```python
from build123d import *

# Parameters (mm, degrees)
SKETCH1_W           = 6.5
SKETCH1_H           = 6.5
SKETCH1_R           = 1.5
BOSS_EXTRUDE1_DEPTH = 5.8
SKETCH2_W           = 6.5
SKETCH2_H           = 5.8
BOSS_EXTRUDE2_DEPTH = 8.85
SKETCH6_W           = 8.85
SKETCH6_H           = 5.8
BOSS_EXTRUDE6_DEPTH = 12.06
SKETCH7_W           = 6.5
SKETCH7_H           = 8.85
BOSS_EXTRUDE7_DEPTH = 75.25
BOSS_EXTRUDE8_DEPTH = 8.85
FILLET3_R           = 20
SKETCH10_R          = 1.125
CUT_EXTRUDE1_DEPTH  = 84.899470201
CUT_EXTRUDE2_START  = -2
SKETCH11_R          = 1.125
CUT_EXTRUDE2_DEPTH  = 2
SKETCH13_W          = 12.06
SKETCH13_H          = 0.25
CUT_EXTRUDE4_DEPTH  = 84.36611182
SKETCH14_W          = 6.5
SKETCH14_H          = 0.25
CUT_EXTRUDE5_DEPTH  = 78.739105989


with BuildPart() as part:
    # Sketch1 → Boss-Extrude1 (new body)
    with BuildSketch(Plane(origin=(0, 0, 0), x_dir=(1, 0, 0), z_dir=(0, 1, 0))):
        Rectangle(SKETCH1_W, SKETCH1_H)
        with Locations(Location((0, 0, 0), (0, 0, 270))):
            Circle(SKETCH1_R, mode=Mode.SUBTRACT)
    extrude(amount=BOSS_EXTRUDE1_DEPTH)

    # Sketch2 → Boss-Extrude2 (add)
    with BuildSketch(Plane.XY.offset(3.25)):
        with Locations((0, 2.9)):
            Rectangle(SKETCH2_W, SKETCH2_H)
    extrude(amount=BOSS_EXTRUDE2_DEPTH)

    # Sketch6 → Boss-Extrude6 (add)
    with BuildSketch(Plane(origin=(3.25, 0, 0), x_dir=(0, 0, -1), z_dir=(1, 0, 0))):
        with Locations((-7.675, 2.9)):
            Rectangle(SKETCH6_W, SKETCH6_H)
    extrude(amount=BOSS_EXTRUDE6_DEPTH)

    # Sketch7 → Boss-Extrude7 (add)
    with BuildSketch(Plane(origin=(0, 5.8, 0), x_dir=(1, 0, 0), z_dir=(0, 1, 0))):
        with Locations((12.06, -7.675)):
            Rectangle(SKETCH7_W, SKETCH7_H)
    extrude(amount=BOSS_EXTRUDE7_DEPTH)

    # Sketch8 → Boss-Extrude8 (add)
    with BuildSketch(Plane.XY.offset(12.1)):
        Polygon((-3.25, 5.8), (8.81, 5.8), (8.81, 17.86), align=None)
    extrude(amount=-BOSS_EXTRUDE8_DEPTH)

    # Fillet3
    fillet3_edges = [part.edges().sort_by_distance(p)[0] for p in [
        (8.81, 17.86, 7.675),
    ]]
    fillet(fillet3_edges, radius=FILLET3_R)

    # Sketch10 → Cut-Extrude1 (cut, through all)
    with BuildSketch(Plane.XY.offset(12.1)):
        with Locations((12.06, 77.25)):
            Circle(SKETCH10_R)
        with Locations((12.06, 40.05)):
            Circle(SKETCH10_R)
    extrude(amount=-CUT_EXTRUDE1_DEPTH, mode=Mode.SUBTRACT)

    # Sketch11 → Cut-Extrude2 (cut)
    # profile 1 of 2: a face of its own
    with BuildSketch(Plane(origin=(0, 0, 3.25), x_dir=(-1, 0, 0), z_dir=(0, 0, -1)).offset(CUT_EXTRUDE2_START)):
        Polygon((-10.111442841, 76.125), (-10.111442841, 78.375), (-12.06, 79.5), (-14.008557159, 78.375), (-14.008557159, 76.125), (-12.06, 75), align=None)
        with Locations(Location((-12.06, 77.25, 0), (0, 0, 180))):
            Circle(SKETCH11_R, mode=Mode.SUBTRACT)
    # profile 2 of 2: a face of its own
    with BuildSketch(Plane(origin=(0, 0, 3.25), x_dir=(-1, 0, 0), z_dir=(0, 0, -1)).offset(CUT_EXTRUDE2_START)):
        Polygon((-10.111442841, 38.925), (-10.111442841, 41.175), (-12.06, 42.3), (-14.008557159, 41.175), (-14.008557159, 38.925), (-12.06, 37.8), align=None)
        with Locations(Location((-12.06, 40.05, 0), (0, 0, 180))):
            Circle(SKETCH11_R, mode=Mode.SUBTRACT)
    extrude(amount=CUT_EXTRUDE2_DEPTH, mode=Mode.SUBTRACT)

    # Sketch13 → Cut-Extrude4 (cut, through all)
    with BuildSketch(Plane(origin=(0, 0, 0), x_dir=(-1, 0, 0), z_dir=(0, -1, 0))):
        with Locations((-9.28, -3.375)):
            Rectangle(SKETCH13_W, SKETCH13_H)
    extrude(amount=-CUT_EXTRUDE4_DEPTH, mode=Mode.SUBTRACT)

    # Sketch14 → Cut-Extrude5 (cut, through all)
    with BuildSketch(Plane(origin=(0, 5.8, 0), x_dir=(1, 0, 0), z_dir=(0, 1, 0))):
        with Locations((0, -3.375)):
            Rectangle(SKETCH14_W, SKETCH14_H)
    extrude(amount=CUT_EXTRUDE5_DEPTH, mode=Mode.SUBTRACT)


solid = part.part
```
Part model, mm, in its own coordinate system. A direction names the side the tool comes from. Round coordinates to 2 decimals unless told otherwise and drop trailing zeros. Write each loop counter-clockwise with the first axis right and the second up, starting at its lowest first coordinate (ties: lowest second). Pieces come first, ordered by that corner, then holes. Notation, with made-up numbers: (2, 81) -> (27, 81) arc R29 ccw to (27, 106) -> close; hole circle Ø11 at (47.25, 45.5). An arc over 180 degrees is marked (long way). Return JSON: item names as keys, results as strings. Group by question number.
Q1. Pin check, flat tips, straight feed: pin 1 (7 mm diameter, centred on y = 50, z = 7, fed in from -X); pin 2 (1.7 mm diameter, centred on y = 2, z = 1, fed in from +X); pin 3 (1.8 mm diameter, centred on x = 12.06, y = 40.05, fed in from +Z); pin 4 (1.5 mm diameter, centred on x = 11.5, y = 53, fed in from -Z). Stop position of each tip, or through.
Q2. Probe L1, parallel to Y at x = 12.06, z = 10 (3 decimals); L2, parallel to X at y = 40.05, z = 9 (3 decimals); L3, parallel to X at y = 1.45, z = 0. List the from-to ranges inside material, lowest first. Write a range as [from, to].
Q3. Saw through at B-B on y = 40.05. Write the cut outline in (x, z) (3 decimals).
Q4. Saw through at C-C on x = -0.75. Write the cut outline in (y, z), plus the area to 3 significant figures.
Q5. Saw through at D-D on z = 0.25. Write the cut outline in (x, y).
Q6. Which spindle directions (+Z, -Z, +X, -X, +Y, -Y) get a long thin tool onto all of the face, cutting with end or side? Do faces 4 (the flat face through (14.009, 40, 4)), 5 (the flat face through (8.81, 53, 8)), 6 (the flat face through (3.25, 3, 0)), 7 (the cylindrical face through (0.45, 2.86, 1.43)). Say none if no direction does.
Q7. Saw through at A-A on z = 7.75. Write the cut outline in (x, y) (3 decimals).
Q8. Mould opens along Y. For faces 1 (the flat face through (10, 31, 3.5)), 2 (the flat face through (0, 5.8, 2)), 3 (the flat face through (14.009, 77, 4)) say: pulls with the +Y half, pulls with the -Y half, needs draft (parallel to the pull), parting line crosses it, or undercut.
Answer:
{
 "1": {"pin 1": "x = 8.81", "pin 2": "x = 3.25", "pin 3": "through", "pin 4": "z = 3.5"},
 "2": {"L1": "[0, 38.925], [41.175, 76.125], [78.375, 81.05]", "L2": "[8.81, 10.935], [13.185, 15.31]", "L3": "[-3.25, -1.5], [1.5, 3.25]"},
 "3": {"outline": "(8.81, 3.5) -> (10.111, 3.5) -> (10.111, 5.25) -> (10.935, 5.25) -> (10.935, 12.1) -> (8.81, 12.1) -> close; (13.185, 5.25) -> (14.009, 5.25) -> (14.009, 3.5) -> (15.31, 3.5) -> (15.31, 12.1) -> (13.185, 12.1) -> close"},
 "4": {"outline": "(0, -3.25) -> (5.8, -3.25) -> (5.8, -1.3) -> (0, -1.3) -> close; (0, 1.3) -> (5.8, 1.3) -> (5.8, 3.5) -> (8.3, 3.5) -> (8.3, 12.1) -> (0, 12.1) -> close", "area": "95.5 mm2"},
 "5": {"outline": "(-3.25, 0) -> (-1.48, 0) -> (-1.48, 5.8) -> (-3.25, 5.8) -> close; (1.48, 0) -> (3.25, 0) -> (3.25, 5.8) -> (1.48, 5.8) -> close"},
 "6": {"face 4": "-Z", "face 5": "+Z, -Z, -X, +Y", "face 6": "-Z, +X, +Y, -Y", "face 7": "+Y, -Y"},
 "7": {"outline": "(-3.25, 0) -> (15.31, 0) -> (15.31, 81.05) -> (8.81, 81.05) -> (8.81, 26.144) arc R20 cw to (2.952, 12.002) -> (-3.25, 5.8) -> close; hole circle Ø2.25 at (12.06, 40.05); hole circle Ø2.25 at (12.06, 77.25)"},
 "8": {"face 1": "needs draft", "face 2": "pulls with the +Y half", "face 3": "undercut"}
}
